```python
from build123d import *

# Parameters (mm, degrees)
SKETCH2_W           = 200
SKETCH2_H           = 150
BOSS_EXTRUDE1_DEPTH = 3
SKETCH3_W           = 200
SKETCH3_H           = 150
SKETCH3_W_2         = 194
SKETCH3_H_2         = 144
BOSS_EXTRUDE2_DEPTH = 50
SKETCH4_W           = 180
SKETCH4_H           = 10
CUT_EXTRUDE3_DEPTH  = 147
SKETCH5_W           = 144
SKETCH5_H           = 7
BOSS_EXTRUDE3_DEPTH = 25
SKETCH6_W           = 144
SKETCH6_H           = 7
BOSS_EXTRUDE4_DEPTH = 25
SKETCH7_W           = 144
SKETCH7_H           = 144
CUT_EXTRUDE5_DEPTH  = 135.629120178
SKETCH8_R           = 3
CUT_EXTRUDE6_DEPTH  = 2
SKETCH9_R           = 1.5
CUT_EXTRUDE7_DEPTH  = 8


with BuildPart() as part:
    # Sketch2 → Boss-Extrude1 (new body)
    with BuildSketch(Plane(origin=(0, 0, 0), x_dir=(1, 0, 0), z_dir=(0, 1, 0))):
        Rectangle(SKETCH2_W, SKETCH2_H)
    extrude(amount=BOSS_EXTRUDE1_DEPTH)

    # Sketch3 → Boss-Extrude2 (add)
    with BuildSketch(Plane(origin=(0, 3, 0), x_dir=(1, 0, 0), z_dir=(0, 1, 0))):
        Rectangle(SKETCH3_W, SKETCH3_H)
        Rectangle(SKETCH3_W_2, SKETCH3_H_2, mode=Mode.SUBTRACT)
    extrude(amount=BOSS_EXTRUDE2_DEPTH)

    # Sketch4 → Cut-Extrude3 (cut)
    with BuildSketch(Plane.XY.offset(75)):
        with Locations((0, 15)):
            Rectangle(SKETCH4_W, SKETCH4_H)
    extrude(amount=-CUT_EXTRUDE3_DEPTH, mode=Mode.SUBTRACT)

    # Sketch5 → Boss-Extrude3 (add)
    with BuildSketch(Plane.ZY.offset(-97)):
        with Locations((0, 6.5)):
            Rectangle(SKETCH5_W, SKETCH5_H)
    extrude(amount=BOSS_EXTRUDE3_DEPTH)

    # Sketch6 → Boss-Extrude4 (add)
    with BuildSketch(Plane(origin=(-97, 0, 0), x_dir=(0, 0, -1), z_dir=(1, 0, 0))):
        with Locations((0, 6.5)):
            Rectangle(SKETCH6_W, SKETCH6_H)
    extrude(amount=BOSS_EXTRUDE4_DEPTH)

    # Sketch7 → Cut-Extrude5 (cut, through all)
    with BuildSketch(Plane(origin=(0, 3, 0), x_dir=(1, 0, 0), z_dir=(0, 1, 0))):
        Rectangle(SKETCH7_W, SKETCH7_H)
    extrude(amount=-CUT_EXTRUDE5_DEPTH, mode=Mode.SUBTRACT)

    # Sketch8 → Cut-Extrude6 (cut)
    with BuildSketch(Plane.XY.offset(75)):
        with Locations((-95, 15)):
            Circle(SKETCH8_R)
        with Locations((95, 15)):
            Circle(SKETCH8_R)
    extrude(amount=-CUT_EXTRUDE6_DEPTH, mode=Mode.SUBTRACT)

    # Sketch9 → Cut-Extrude7 (cut)
    with BuildSketch(Plane.XZ):
        with Locations(Location((-95, 70, 0), (0, 0, 270))):
            Circle(SKETCH9_R)
        with Locations(Location((95, 70, 0), (0, 0, 270))):
            Circle(SKETCH9_R)
        with Locations(Location((95, -70, 0), (0, 0, 270))):
            Circle(SKETCH9_R)
        with Locations(Location((-95, -70, 0), (0, 0, 270))):
            Circle(SKETCH9_R)
    extrude(amount=-CUT_EXTRUDE7_DEPTH, mode=Mode.SUBTRACT)


solid = part.part
```
For this review, take the finished solid that the model builds, in its own axes (mm). A direction names the side the tool comes from. Coordinates: 2 decimals unless noted, no trailing zeros. Order: outer loops, then holes, each group sorted by start corner. A loop starts at its lowest first (then second) coordinate and runs counter-clockwise, first axis right, second up. Notation, with made-up numbers: (81.5, 78) - (116.5, 78) arc R27 ccw to (116.5, 112) - close; hole circle Ø5 at (71, 12). An arc over 180 degrees is marked (long way). Answer as a JSON object with one key per item and string values. Group by question number.
1. Clearance check with flat-ended pins moving along their axes: P1, Ø2.5, axis at x = 95, z = -70, coming from the +Y side; P2, Ø3.5, axis at x = 95, y = 15, coming from the +Z side; P3, Ø3, axis at x = -64.5, y = 12, coming from the +Z side. State where each tip first meets the part, or that it passes through.
2. We need section D-D on x = 61.5. State the section outline as (y, z) points.
3. The part is to be moulded in two halves that separate along X. For faces 5 (the flat face through (100, 26, 1)), 6 (the flat face through (0, 53, -73)), 7 (the flat face through (-1, 36, 72)), say which applies: pulls with the +X half, pulls with the -X half, needs draft (parallel to the pull), parting line crosses it, or undercut.
4. For probe 1 along X at (y, z) = (2.5, 70); probe 2 along Z at (x, y) = (95, 2); probe 3 along X at (y, z) = (50, 65.5), list the stretches that pass through material, from the lowest coordinate up.
5. For faces 1 (the flat face through (-1, 5, 72)), 2 (the flat face through (-8, 10, 73)), 3 (the flat face through (-97, 31, 1)), 4 (the flat face through (-95, 15, 73)), list the 3-axis set-ups (+Z, -Z, +X, -X, +Y, -Y) from which the entire face can be reached by the end or side of a thin tool; tool diameter is ignored.
6. We need section B-B on x = -85. State the section outline as (y, z) points, then the cut area to 3 significant figures.
7. We need section C-C on y = 4.5. State the section outline as (x, z) points.
8. We need section A-A on z = -1. State the section outline as (x, y) points.
Final values:
{
 "1": {"P1": "y = 10", "P2": "z = 73", "P3": "z = -72"},
 "2": {"outline": "(0, -75) - (53, -75) - (53, -72) - (0, -72) - close; (0, 72) - (10, 72) - (10, 75) - (0, 75) - close; (20, 72) - (53, 72) - (53, 75) - (20, 75) - close"},
 "3": {"face 5": "pulls with the +X half", "face 6": "needs draft", "face 7": "undercut"},
 "4": {"probe 1": "-100 to -96.5, -93.5 to -72, 72 to 93.5, 96.5 to 100", "probe 2": "-75 to -71.5, -68.5 to 68.5, 71.5 to 75", "probe 3": "-100 to -97, 97 to 100"},
 "5": {"face 1": "+Y, -Y", "face 2": "none", "face 3": "+Y", "face 4": "+Z"},
 "6": {"outline": "(0, -75) - (53, -75) - (53, -72) - (10, -72) - (10, 75) - (0, 75) - close; (20, 72) - (53, 72) - (53, 75) - (20, 75) - close", "area": "1,730 mm²"},
 "7": {"outline": "(-100, -75) - (100, -75) - (100, 75) - (-100, 75) - close; hole circle Ø3 at (-95, -70); hole circle Ø3 at (-95, 70); hole (-72, -72) - (72, -72) - (72, 72) - (-72, 72) - close; hole circle Ø3 at (95, -70); hole circle Ø3 at (95, 70)"},
 "8": {"outline": "(-100, 0) - (-72, 0) - (-72, 10) - (-97, 10) - (-97, 53) - (-100, 53) - close; (72, 0) - (100, 0) - (100, 53) - (97, 53) - (97, 10) - (72, 10) - close"}
}
